from build123d import *

# Parameters (mm, degrees)
BOSS_EXTRUDE1_DEPTH  = 25.5
CUT_EXTRUDE1_DEPTH   = 26.12
LPATTERN1_COUNT      = 4
LPATTERN1_PITCH      = 4.5
LPATTERN1_COUNT_DIR2 = 9
LPATTERN1_PITCH_DIR2 = 4.5


with BuildPart() as part:
    # Sketch1 → Boss-Extrude1 (new body)
    with BuildSketch(Plane.XY):
        Polygon((-14.215030011, 7), (-14.215030011, -0.249149017), (0.939234275, -0.249149017), (3.390192413, -0.249149017), (3.390192413, 7), align=None)
    extrude(amount=BOSS_EXTRUDE1_DEPTH)

    # Sketch2 → Cut-Extrude1 (cut)
    with BuildSketch(Plane.XY):
        with BuildLine():
            ThreePointArc((-6.881285782, 3.348371163), (-7.417069895, 3.826658598), (-7.671285782, 4.498371163))
            ThreePointArc((-7.671285782, 4.498371163), (-7.912320341, 6.04482582), (-8.981285782, 7.188037328))
            ThreePointArc((-8.981285782, 7.188037328), (-6.881285782, 7.762283268), (-4.781285782, 7.188037328))
            ThreePointArc((-4.781285782, 7.188037328), (-5.850251222, 6.04482582), (-6.091285782, 4.498371163))
            ThreePointArc((-6.091285782, 4.498371163), (-6.345501668, 3.826658598), (-6.881285782, 3.348371163))
        make_face()
    cut_extrude1 = extrude(amount=CUT_EXTRUDE1_DEPTH, mode=Mode.SUBTRACT)

    # LPattern1: Cut-Extrude1 4 × 9
    with Locations(*[Vector(-1, 0, 0) * (i * LPATTERN1_PITCH) + Vector(1, 0, 0) * (j * LPATTERN1_PITCH_DIR2) for i in range(LPATTERN1_COUNT) for j in range(LPATTERN1_COUNT_DIR2) if (i, j) != (0, 0)]):
        add(cut_extrude1, mode=Mode.SUBTRACT)


solid = part.part
Geometry check sheet. Reference: the model listing, model coordinates, mm. A direction names the side the tool comes from. Round coordinates to 2 decimals unless told otherwise and drop trailing zeros. Order: outer loops, then holes, each group sorted by start corner. A loop starts at its lowest first (then second) coordinate and runs counter-clockwise, first axis right, second up. Notation, with made-up numbers: M 27,31.5 L 50,31.5 A16 cw 50,47.5 Z; hole C -10,20.25 d7. An arc over 180 degrees is marked long. Write each question's results on one line, items separated by ' | '. Start each with the question number.
1. Set-up check for faces 1 (the face through (2.96, 5.53, 12.57)), 2 (the face through (-6, 3, 0)): record each of +Z, -Z, +X, -X, +Y, -Y from which the full face is reachable in a straight line by a thin tool's end or side.
2. Material ranges on L1, parallel to X at y = 4.5, z = 17; L2, parallel to X at y = 5, z = 22.25; L3, parallel to X at y = 6.75, z = 11, recorded low to high. Write a range as from..to.
3. Draft check along X on faces 3 (the face through (-14.215, 3, 13)), 4 (the face through (-6, -0.249, 13)), 5 (the face through (-7.4, 3.8, 12.6)). Enter one of: pulls with the +X half, pulls with the -X half, needs draft (parallel to the pull), parting line crosses it, or undercut.
4. Cross-section at B-B on x = -1.25. Record the boundary of the cut face in (y, z), plus the area to 3 significant figures.
5. Cross-section at A-A on z = 22. Record the boundary of the cut face in (x, y), plus the area to 3 significant figures.
6. Cross-section at C-C on x = 0.75. Record the boundary of the cut face in (y, z), plus the area to 3 significant figures.
Resolved:
1) face 1: +Z, -Z | face 2: -Z, +X, -X, +Y, -Y
2) L1: -14.22..-12.17, -10.59..-7.67, -6.09..-3.17, -1.59..1.33, 2.91..3.39 | L2: -14.22..-12.15, -10.62..-7.65, -6.12..-3.15, -1.62..1.35, 2.88..3.39 | L3: -14.22..-12.91, -9.85..-8.41, -5.35..-3.91, -0.85..0.59
3) face 3: pulls with the -X half | face 4: needs draft | face 5: undercut
4) outline: M -0.25,0 L 6.23,0 L 6.23,25.5 L -0.25,25.5 Z | area: 165 mm2
5) outline: M -14.22,-0.25 L 3.39,-0.25 L 3.39,6.44 A2.66 ccw 2.91,4.5 A1.51 cw 2.12,3.35 A1.51 cw 1.33,4.5 A2.66 ccw 0.3,7 L -0.57,7 A2.66 ccw -1.59,4.5 A1.51 cw -2.38,3.35 A1.51 cw -3.17,4.5 A2.66 ccw -4.2,7 L -5.07,7 A2.66 ccw -6.09,4.5 A1.51 cw -6.88,3.35 A1.51 cw -7.67,4.5 A2.66 ccw -8.7,7 L -9.57,7 A2.66 ccw -10.59,4.5 A1.51 cw -11.38,3.35 A1.51 cw -12.17,4.5 A2.66 ccw -13.2,7 L -14.07,7 A2.66 ccw -14.22,6.88 Z | area: 102 mm2
6) outline: M -0.25,0 L 6.57,0 L 6.57,25.5 L -0.25,25.5 Z | area: 174 mm2
